Read the model definition and answer for the solid it produces. Units are mm, in the model's axes. Give positions to 0.01 mm unless a question says otherwise; leave off trailing zeros. Order: outer loops, then holes, each group sorted by start corner. A loop starts at its lowest first (then second) coordinate and runs counter-clockwise, first axis right, second up. Notation, with made-up numbers: (27, 43) - (81, 43) arc R13 ccw to (81, 53) - close; hole circle Ø6 at (35.25, -2). An arc over 180 degrees is marked (long way). Write each question's results on one line, items separated by ' | '.
from build123d import *

# Parameters (mm, degrees)
SKETCH1_W           = 70
SKETCH1_H           = 85
BOSS_EXTRUDE1_DEPTH = 4
SKETCH2_R           = 2.85
SKETCH2_R_2         = 19.25
CUT_EXTRUDE1_DEPTH  = 56.201902141
FILLET1_R           = 3


with BuildPart() as part:
    # Sketch1 → Boss-Extrude1 (new body)
    with BuildSketch(Plane(origin=(0, 0, 0), x_dir=(1, 0, 0), z_dir=(0, 1, 0))):
        Rectangle(SKETCH1_W, SKETCH1_H)
    extrude(amount=BOSS_EXTRUDE1_DEPTH)

    # Sketch2 → Cut-Extrude1 (cut, through all)
    with BuildSketch(Plane(origin=(0, 4, 0), x_dir=(1, 0, 0), z_dir=(0, 1, 0))):
        with Locations(Location((-23.57, 11.07, 0), (0, 0, 270))):
            Circle(SKETCH2_R)
        with Locations(Location((-23.57, -36.07, 0), (0, 0, 270))):
            Circle(SKETCH2_R)
        with Locations(Location((23.57, -36.07, 0), (0, 0, 270))):
            Circle(SKETCH2_R)
        with Locations(Location((23.57, 11.07, 0), (0, 0, 270))):
            Circle(SKETCH2_R)
        with Locations(Location((0, -12.5, 0), (0, 0, 270))):
            Circle(SKETCH2_R_2)
        with Locations(Location((15, 31.5, 0), (0, 0, 270))):
            Circle(SKETCH2_R)
        with Locations(Location((-15, 31.5, 0), (0, 0, 270))):
            Circle(SKETCH2_R)
    extrude(amount=-CUT_EXTRUDE1_DEPTH, mode=Mode.SUBTRACT)

    # Fillet1
    fillet1_edges = [part.edges().sort_by_distance(p)[0] for p in [
        (35, 2, 42.5),
        (-35, 2, 42.5),
    ]]
    fillet(fillet1_edges, radius=FILLET1_R)


solid = part.part
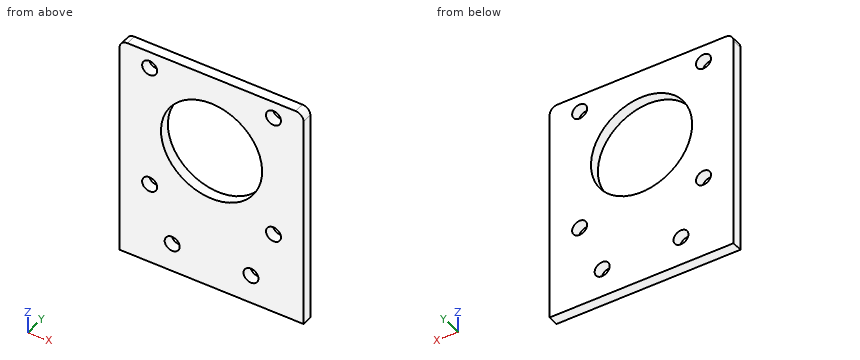
(1) Section A-A (z = 12.5) is taken. Give the vertices of the cut face in (x, y).
Conclusion:
outline: (-35, 0) - (-19.25, 0) - (-19.25, 4) - (-35, 4) - close; (19.25, 0) - (35, 0) - (35, 4) - (19.25, 4) - close
(2) Section B-B (x = -23.57) is taken. Give the vertices of the cut face in (y, z).
Conclusion:
outline: (0, -42.5) - (4, -42.5) - (4, -13.92) - (0, -13.92) - close; (0, -8.22) - (4, -8.22) - (4, 33.22) - (0, 33.22) - close; (0, 38.92) - (4, 38.92) - (4, 42.5) - (0, 42.5) - close
(3) Section D-D (y = 1.05) is taken. Give the vertices of the cut face in (x, z), plus the area to 3 significant figures.
Conclusion:
outline: (-35, -42.5) - (35, -42.5) - (35, 39.5) arc R3 ccw to (32, 42.5) - (-32, 42.5) arc R3 ccw to (-35, 39.5) - close; hole circle Ø5.7 at (-23.57, -11.07); hole circle Ø5.7 at (-23.57, 36.07); hole circle Ø38.5 at (0, 12.5); hole circle Ø5.7 at (-15, -31.5); hole circle Ø5.7 at (15, -31.5); hole circle Ø5.7 at (23.57, -11.07); hole circle Ø5.7 at (23.57, 36.07) | area: 4,630 mm^2
(4) Section C-C (z = 36.07) is taken. Give the vertices of the cut face in (x, y), plus the area to 3 significant figures.
Conclusion:
outline: (-35, 0) - (-26.42, 0) - (-26.42, 4) - (-35, 4) - close; (-20.72, 0) - (20.72, 0) - (20.72, 4) - (-20.72, 4) - close; (26.42, 0) - (35, 0) - (35, 4) - (26.42, 4) - close | area: 234 mm^2
(5) Consider probe 1 along X at (y, z) = (2.6, -31.5); probe 2 along X at (y, z) = (2.1, 36.07); probe 3 along Z at (x, y) = (22, 0.25). Determine where each line is inside the solid, lowest interval first. Write a range as [from, to].
Conclusion:
probe 1: [-35, -17.85], [-12.15, 12.15], [17.85, 35] | probe 2: [-35, -26.42], [-20.72, 20.72], [26.42, 35] | probe 3: [-42.5, -13.45], [-8.69, 33.69], [38.45, 42.5]
